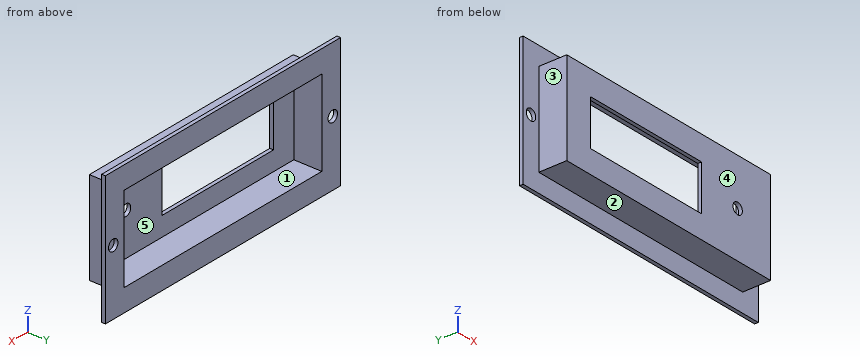
from build123d import *

# Parameters (mm, degrees)
CROQUIS1_W              = 130
CROQUIS1_H              = 50
SALIENTE_EXTRUIR1_DEPTH = 30
CROQUIS2_W              = 126
CROQUIS2_H              = 46
CORTAR_EXTRUIR1_DEPTH   = 28
CROQUIS3_R              = 3
CROQUIS3_W              = 70.999999967
CROQUIS3_H              = 24.5
CORTAR_EXTRUIR2_DEPTH   = 2
CROQUIS9_W              = 150
CROQUIS9_H              = 70
CROQUIS9_W_2            = 130
CROQUIS9_H_2            = 50
SALIENTE_EXTRUIR3_DEPTH = 15
CROQUIS9_2_W            = 150
CROQUIS9_2_H            = 70
CROQUIS9_2_W_2          = 130
CROQUIS9_2_H_2          = 50
CORTAR_EXTRUIR5_DEPTH   = 13
CROQUIS11_R             = 3
CORTAR_EXTRUIR6_DEPTH   = 2
CROQUIS12_W             = 50
CROQUIS12_H             = 13
CORTAR_EXTRUIR7_DEPTH   = 130


with BuildPart() as part:
    # Croquis1 → Saliente-Extruir1 (new body)
    with BuildSketch(Plane(origin=(0, 0, 0), x_dir=(1, 0, 0), z_dir=(0, 1, 0))):
        Rectangle(CROQUIS1_W, CROQUIS1_H)
    extrude(amount=SALIENTE_EXTRUIR1_DEPTH)

    # Croquis2 → Cortar-Extruir1 (cut)
    with BuildSketch(Plane(origin=(0, 30, 0), x_dir=(1, 0, 0), z_dir=(0, 1, 0))):
        Rectangle(CROQUIS2_W, CROQUIS2_H)
    extrude(amount=-CORTAR_EXTRUIR1_DEPTH, mode=Mode.SUBTRACT)

    # Croquis3 → Cortar-Extruir2 (cut)
    with BuildSketch(Plane.XZ):
        with Locations(Location((43.9980881, -0.173527089, 0), (0, 0, 270))):
            Circle(CROQUIS3_R)
        with Locations((-14.500000016, -0.45006101)):
            Rectangle(CROQUIS3_W, CROQUIS3_H)
    extrude(amount=-CORTAR_EXTRUIR2_DEPTH, mode=Mode.SUBTRACT)

    # Croquis9 → Saliente-Extruir3 (add)
    with BuildSketch(Plane(origin=(0, 30, 0), x_dir=(1, 0, 0), z_dir=(0, 1, 0))):
        Rectangle(CROQUIS9_W, CROQUIS9_H)
        Rectangle(CROQUIS9_W_2, CROQUIS9_H_2, mode=Mode.SUBTRACT)
    extrude(amount=-SALIENTE_EXTRUIR3_DEPTH)

    # Croquis9<2> → Cortar-Extruir5 (cut)
    with BuildSketch(Plane(origin=(0, 30, 0), x_dir=(1, 0, 0), z_dir=(0, 1, 0))):
        Rectangle(CROQUIS9_2_W, CROQUIS9_2_H)
        Rectangle(CROQUIS9_2_W_2, CROQUIS9_2_H_2, mode=Mode.SUBTRACT)
    extrude(amount=-CORTAR_EXTRUIR5_DEPTH, mode=Mode.SUBTRACT)

    # Croquis11 → Cortar-Extruir6 (cut)
    with BuildSketch(Plane(origin=(0, 17, 0), x_dir=(1, 0, 0), z_dir=(0, 1, 0))):
        with Locations(Location((-70, 0, 0), (0, 0, 270))):
            Circle(CROQUIS11_R)
        with Locations(Location((70, 0, 0), (0, 0, 270))):
            Circle(CROQUIS11_R)
    extrude(amount=-CORTAR_EXTRUIR6_DEPTH, mode=Mode.SUBTRACT)

    # Croquis12 → Cortar-Extruir7 (cut)
    with BuildSketch(Plane.ZY.offset(65)):
        with Locations((0, 23.5)):
            Rectangle(CROQUIS12_W, CROQUIS12_H)
    extrude(amount=-CORTAR_EXTRUIR7_DEPTH, mode=Mode.SUBTRACT)


solid = part.part
The model under review builds one solid part; all positions refer to its coordinate system, in mm. Face numbers are marked on the shaded views. A direction names the side the tool comes from. Give positions to 0.01 mm unless a question says otherwise; leave off trailing zeros. Order: outer loops, then holes, each group sorted by start corner. A loop starts at its lowest first (then second) coordinate and runs counter-clockwise, first axis right, second up. Notation, with made-up numbers: M -20.75,31.25 L 37.25,31.25 A20 ccw 37.25,38.25 Z; hole C -15,24 d3. An arc over 180 degrees is marked long. Answer in a Markdown table with one row per item. Add a question column.
1. To check wall thickness, follow line 1 along X through (y, z) = (15.75, 0); line 2 along Z through (x, y) = (51, 6); line 3 along X through (y, z) = (9.75, 0). State the ranges of each line that lie inside material, in increasing order.
2. Add section C-C on y = 8. State the section outline as (x, z) points.
3. For pin 1 Ø4.5 at (x, y) = (8, 11) entering from -Z; pin 2 Ø1 at (x, y) = (0.5, 0.5) entering from +Z; pin 3 Ø4 at (y, z) = (6.5, 3.5) entering from -X; pin 4 Ø5.5 at (x, z) = (-70, 0) entering from -Y, all flat-tipped, find the tip position at first contact; note any pin that passes through.
4. Machinability: for the marked faces 4 and 5, which of the approach directions +Z, -Z, +X, -X, +Y, -Y give a long, thin tool a straight path to every point of the face, cutting with its end or side? Answer none if there is none.
5. Mouldability with a two-part tool opening along X and no side actions: class the marked faces 1, 2 and 3 as released by +X, released by -X, zero draft, split by the parting line, or undercut.
6. Add section B-B on z = 8.5. State the section outline as (x, y) points.
7. Add section A-A on x = -70. State the section outline as (y, z) points.
8. Add section D-D on z = 15.5. State the section outline as (x, y) points, plus the area to 3 significant figures.
The answers:
| question | item | result |
|---|---|---|
| 1 | line 1 | -75 to -73, -67 to -63, 63 to 67, 73 to 75 |
| 1 | line 2 | -25 to -23, 23 to 25 |
| 1 | line 3 | -65 to -63, 63 to 65 |
| 2 | outline | M -65,-25 L 65,-25 L 65,25 L -65,25 Z; hole M -63,-23 L 63,-23 L 63,23 L -63,23 Z |
| 3 | pin 1 | z = -25 |
| 3 | pin 2 | z = 25 |
| 3 | pin 3 | x = -65 |
| 3 | pin 4 | through |
| 4 | face 4 | +Z, -Z, +X, -X, -Y |
| 4 | face 5 | +Y |
| 5 | face 1 | undercut |
| 5 | face 2 | zero draft |
| 5 | face 3 | released by -X |
| 6 | outline | M -75,15 L -65,15 L -65,0 L -50,0 L -50,2 L -63,2 L -63,17 L -75,17 Z; M 21,0 L 65,0 L 65,15 L 75,15 L 75,17 L 63,17 L 63,2 L 21,2 Z |
| 7 | outline | M 15,-35 L 17,-35 L 17,-3 L 15,-3 Z; M 15,3 L 17,3 L 17,35 L 15,35 Z |
| 8 | outline | M -75,15 L -65,15 L -65,0 L 65,0 L 65,15 L 75,15 L 75,17 L 63,17 L 63,2 L -63,2 L -63,17 L -75,17 Z |
| 8 | area | 360 mm2 |
